Geometry: final body of the model. Coordinates: model frame, mm. Face numbers are marked on the shaded views. A direction names the side the tool comes from. Round coordinates to 2 decimals unless told otherwise and drop trailing zeros. Loops run counter-clockwise (first coordinate to the right, second up) from the corner with the lowest first, then second, coordinate; pieces in that order, holes last. Notation, with made-up numbers: M -25.5,82 L -8.5,82 A13 cw -8.5,92 Z; hole C 44.5,36 d8. An arc over 180 degrees is marked long. Write each question's results on one line, items separated by ' | '.
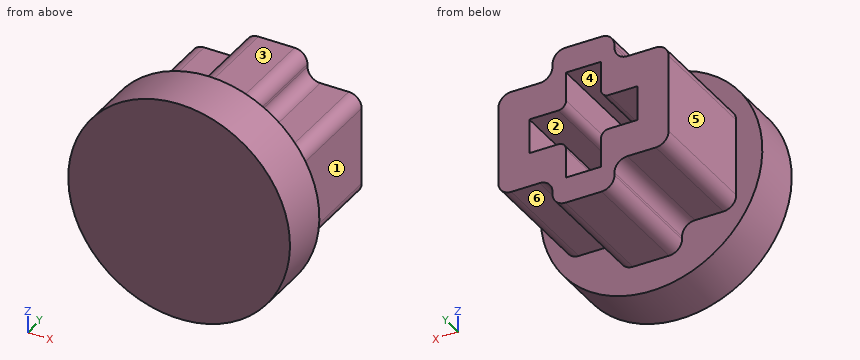
```python
from build123d import *

# Parameters (mm, degrees)
BUTTON_TOP_DEPTH        = 1.8
BUTTON_WALLS_DEPTH      = 4.8
OFFSET_2_DEPTH          = 0.2
STEM_START              = 0.2
STEM_HOUSING_DEPTH      = 4.6
SPOKES_DEPTH            = 0.2
CHAMFER1_SIZE           = 1.5
SKETCH11_R              = 47.776797093
SKETCH11_R_2            = 4.295081168
CUT_EXTRUDE1_DEPTH      = 10
CUT_EXTRUDE1_DEPTH_BACK = 10


with BuildPart() as part:
    # Sketch1 → button top (new body)
    with BuildSketch(Plane(origin=(0, 0, 0), x_dir=(1, 0, 0), z_dir=(0, 1, 0))):
        with BuildLine():
            Line((17, -12), (-17, -12))
            ThreePointArc((-17, -12), (-29, 0), (-17, 12))
            Line((-17, 12), (17, 12))
            ThreePointArc((17, 12), (29, 0), (17, -12))
        make_face()
    extrude(amount=BUTTON_TOP_DEPTH)

    # Sketch2 → button walls (add)
    with BuildSketch(Plane(origin=(0, 1.8, 0), x_dir=(1, 0, 0), z_dir=(0, 1, 0))):
        with BuildLine():
            Line((-17, 12), (17, 12))
            ThreePointArc((17, 12), (29, 0), (17, -12))
            Line((17, -12), (-17, -12))
            ThreePointArc((-17, -12), (-29, 0), (-17, 12))
        make_face()
        with BuildLine():
            Line((-17, 10.2), (17, 10.2))
            ThreePointArc((17, 10.2), (27.2, 0), (17, -10.2))
            Line((17, -10.2), (-17, -10.2))
            ThreePointArc((-17, -10.2), (-27.2, 0), (-17, 10.2))
        make_face(mode=Mode.SUBTRACT)
    extrude(amount=BUTTON_WALLS_DEPTH)

    # Sketch5 → offset 2 (add)
    with BuildSketch(Plane(origin=(0, 1.8, 0), x_dir=(1, 0, 0), z_dir=(0, 1, 0))):
        with BuildLine():
            Line((-12, 5), (12, 5))
            ThreePointArc((12, 5), (17, 0), (12, -5))
            Line((12, -5), (-12, -5))
            ThreePointArc((-12, -5), (-17, 0), (-12, 5))
        make_face()
    extrude(amount=OFFSET_2_DEPTH)

    # Sketch3 → stem housing (add)
    with BuildSketch(Plane(origin=(0, 1.8, 0), x_dir=(1, 0, 0), z_dir=(0, 1, 0)).offset(STEM_START)):
        with BuildLine():
            Line((-3.6, 2.6), (-3.6, -2.6))
            Line((-3.6, -2.6), (-1.496662955, -2.6))
            ThreePointArc((-1.496662955, -2.6), (0, -3), (1.496662955, -2.6))
            Line((1.496662955, -2.6), (3.6, -2.6))
            Line((3.6, -2.6), (3.6, 2.6))
            Line((3.6, 2.6), (1.496662955, 2.6))
            ThreePointArc((1.496662955, 2.6), (0, 3), (-1.496662955, 2.6))
            Line((-1.496662955, 2.6), (-3.6, 2.6))
        make_face()
        with BuildLine():
            Line((-0.675, 0.975), (-0.675, 2.1))
            Line((-0.675, 2.1), (0.675, 2.1))
            Line((0.675, 2.1), (0.675, 0.975))
            ThreePointArc((0.675, 0.975), (0.762867966, 0.762867966), (0.975, 0.675))
            Line((0.975, 0.675), (2.1, 0.675))
            Line((2.1, 0.675), (2.1, -0.675))
            Line((2.1, -0.675), (0.975, -0.675))
            ThreePointArc((0.975, -0.675), (0.762867966, -0.762867966), (0.675, -0.975))
            Line((0.675, -0.975), (0.675, -2.1))
            Line((0.675, -2.1), (-0.675, -2.1))
            Line((-0.675, -2.1), (-0.675, -0.975))
            ThreePointArc((-0.675, -0.975), (-0.762867966, -0.762867966), (-0.975, -0.675))
            Line((-0.975, -0.675), (-2.1, -0.675))
            Line((-2.1, -0.675), (-2.1, 0.675))
            Line((-2.1, 0.675), (-0.975, 0.675))
            ThreePointArc((-0.975, 0.675), (-0.762867966, 0.762867966), (-0.675, 0.975))
        make_face(mode=Mode.SUBTRACT)
        with BuildLine():
            ThreePointArc((14.738, -2), (15.091553391, -1.853553391), (15.238, -1.5))
            Line((15.238, -1.5), (15.238, 1.5))
            ThreePointArc((15.238, 1.5), (15.091553391, 1.853553391), (14.738, 2))
            Line((14.738, 2), (13.638, 2))
            ThreePointArc((13.638, 2), (13.284446609, 2.146446609), (13.138, 2.5))
            Line((13.138, 2.5), (13.138, 2.6))
            ThreePointArc((13.138, 2.6), (12.991553391, 2.953553391), (12.638, 3.1))
            Line((12.638, 3.1), (11.238, 3.1))
            ThreePointArc((11.238, 3.1), (10.884446609, 2.953553391), (10.738, 2.6))
            Line((10.738, 2.6), (10.738, 2.5))
            ThreePointArc((10.738, 2.5), (10.591553391, 2.146446609), (10.238, 2))
            Line((10.238, 2), (9.138, 2))
            ThreePointArc((9.138, 2), (8.784446609, 1.853553391), (8.638, 1.5))
            Line((8.638, 1.5), (8.638, -1.5))
            ThreePointArc((8.638, -1.5), (8.784446609, -1.853553391), (9.138, -2))
            Line((9.138, -2), (10.238, -2))
            ThreePointArc((10.238, -2), (10.591553391, -2.146446609), (10.738, -2.5))
            Line((10.738, -2.5), (10.738, -2.6))
            ThreePointArc((10.738, -2.6), (10.884446609, -2.953553391), (11.238, -3.1))
            Line((11.238, -3.1), (12.638, -3.1))
            ThreePointArc((12.638, -3.1), (12.991553391, -2.953553391), (13.138, -2.6))
            Line((13.138, -2.6), (13.138, -2.5))
            ThreePointArc((13.138, -2.5), (13.284446609, -2.146446609), (13.638, -2))
            Line((13.638, -2), (14.738, -2))
        make_face()
        with BuildLine():
            Line((14.038, 0.675), (14.038, -0.675))
            Line((14.038, -0.675), (12.913, -0.675))
            ThreePointArc((12.913, -0.675), (12.700867966, -0.762867966), (12.613, -0.975))
            Line((12.613, -0.975), (12.613, -2.1))
            Line((12.613, -2.1), (11.263, -2.1))
            Line((11.263, -2.1), (11.263, -0.975))
            ThreePointArc((11.263, -0.975), (11.175132034, -0.762867966), (10.963, -0.675))
            Line((10.963, -0.675), (9.838, -0.675))
            Line((9.838, -0.675), (9.838, 0.675))
            Line((9.838, 0.675), (10.963, 0.675))
            ThreePointArc((10.963, 0.675), (11.175132034, 0.762867966), (11.263, 0.975))
            Line((11.263, 0.975), (11.263, 2.1))
            Line((11.263, 2.1), (12.613, 2.1))
            Line((12.613, 2.1), (12.613, 0.975))
            ThreePointArc((12.613, 0.975), (12.700867966, 0.762867966), (12.913, 0.675))
            Line((12.913, 0.675), (14.038, 0.675))
        make_face(mode=Mode.SUBTRACT)
        with BuildLine():
            Line((-13.138, 2.6), (-13.138, 2.5))
            ThreePointArc((-13.138, 2.5), (-13.284446609, 2.146446609), (-13.638, 2))
            Line((-13.638, 2), (-14.738, 2))
            ThreePointArc((-14.738, 2), (-15.091553391, 1.853553391), (-15.238, 1.5))
            Line((-15.238, 1.5), (-15.238, -1.5))
            ThreePointArc((-15.238, -1.5), (-15.091553391, -1.853553391), (-14.738, -2))
            Line((-14.738, -2), (-13.638, -2))
            ThreePointArc((-13.638, -2), (-13.284446609, -2.146446609), (-13.138, -2.5))
            Line((-13.138, -2.5), (-13.138, -2.6))
            ThreePointArc((-13.138, -2.6), (-12.991553391, -2.953553391), (-12.638, -3.1))
            Line((-12.638, -3.1), (-11.238, -3.1))
            ThreePointArc((-11.238, -3.1), (-10.884446609, -2.953553391), (-10.738, -2.6))
            Line((-10.738, -2.6), (-10.738, -2.5))
            ThreePointArc((-10.738, -2.5), (-10.591553391, -2.146446609), (-10.238, -2))
            Line((-10.238, -2), (-9.138, -2))
            ThreePointArc((-9.138, -2), (-8.784446609, -1.853553391), (-8.638, -1.5))
            Line((-8.638, -1.5), (-8.638, 1.5))
            ThreePointArc((-8.638, 1.5), (-8.784446609, 1.853553391), (-9.138, 2))
            Line((-9.138, 2), (-10.238, 2))
            ThreePointArc((-10.238, 2), (-10.591553391, 2.146446609), (-10.738, 2.5))
            Line((-10.738, 2.5), (-10.738, 2.6))
            ThreePointArc((-10.738, 2.6), (-10.884446609, 2.953553391), (-11.238, 3.1))
            Line((-11.238, 3.1), (-12.638, 3.1))
            ThreePointArc((-12.638, 3.1), (-12.991553391, 2.953553391), (-13.138, 2.6))
        make_face()
        with BuildLine():
            ThreePointArc((-12.913, 0.675), (-12.700867966, 0.762867966), (-12.613, 0.975))
            Line((-12.613, 0.975), (-12.613, 2.1))
            Line((-12.613, 2.1), (-11.263, 2.1))
            Line((-11.263, 2.1), (-11.263, 0.975))
            ThreePointArc((-11.263, 0.975), (-11.175132034, 0.762867966), (-10.963, 0.675))
            Line((-10.963, 0.675), (-9.838, 0.675))
            Line((-9.838, 0.675), (-9.838, -0.675))
            Line((-9.838, -0.675), (-10.963, -0.675))
            ThreePointArc((-10.963, -0.675), (-11.175132034, -0.762867966), (-11.263, -0.975))
            Line((-11.263, -0.975), (-11.263, -2.1))
            Line((-11.263, -2.1), (-12.613, -2.1))
            Line((-12.613, -2.1), (-12.613, -0.975))
            ThreePointArc((-12.613, -0.975), (-12.700867966, -0.762867966), (-12.913, -0.675))
            Line((-12.913, -0.675), (-14.038, -0.675))
            Line((-14.038, -0.675), (-14.038, 0.675))
            Line((-14.038, 0.675), (-12.913, 0.675))
        make_face(mode=Mode.SUBTRACT)
    extrude(amount=STEM_HOUSING_DEPTH)

    # Sketch4 → spokes (add)
    with BuildSketch(Plane(origin=(0, 1.8, 0), x_dir=(1, 0, 0), z_dir=(0, 1, 0))):
        with BuildLine():
            Line((-0.8, 3), (-0.8, 10.2))
            ThreePointArc((-0.8, 10.2), (0, 11), (0.8, 10.2))
            Line((0.8, 10.2), (0.8, 3))
            ThreePointArc((0.8, 3), (0, 2.2), (-0.8, 3))
        make_face()
        with BuildLine():
            Line((17, -0.8), (27.2, -0.8))
            ThreePointArc((27.2, -0.8), (28, 0), (27.2, 0.8))
            Line((27.2, 0.8), (17, 0.8))
            ThreePointArc((17, 0.8), (16.2, 0), (17, -0.8))
        make_face()
        with BuildLine():
            Line((11.2, 3.1), (11.2, 10.2))
            ThreePointArc((11.2, 10.2), (12, 11), (12.8, 10.2))
            Line((12.8, 10.2), (12.8, 3.1))
            ThreePointArc((12.8, 3.1), (12, 2.3), (11.2, 3.1))
        make_face()
        with BuildLine():
            Line((-12.8, 3.1), (-12.8, 10.2))
            ThreePointArc((-12.8, 10.2), (-12, 11), (-11.2, 10.2))
            Line((-11.2, 10.2), (-11.2, 3.1))
            ThreePointArc((-11.2, 3.1), (-12, 2.3), (-12.8, 3.1))
        make_face()
        with BuildLine():
            Line((-17, -0.8), (-27.2, -0.8))
            ThreePointArc((-27.2, -0.8), (-28, 0), (-27.2, 0.8))
            Line((-27.2, 0.8), (-17, 0.8))
            ThreePointArc((-17, 0.8), (-16.2, 0), (-17, -0.8))
        make_face()
        with BuildLine():
            Line((-0.8, -3), (-0.8, -10.2))
            ThreePointArc((-0.8, -10.2), (0, -11), (0.8, -10.2))
            Line((0.8, -10.2), (0.8, -3))
            ThreePointArc((0.8, -3), (0, -2.2), (-0.8, -3))
        make_face()
        with BuildLine():
            Line((11.2, -3.1), (11.2, -10.2))
            ThreePointArc((11.2, -10.2), (12, -11), (12.8, -10.2))
            Line((12.8, -10.2), (12.8, -3.1))
            ThreePointArc((12.8, -3.1), (12, -2.3), (11.2, -3.1))
        make_face()
        with BuildLine():
            Line((-12.8, -3.1), (-12.8, -10.2))
            ThreePointArc((-12.8, -10.2), (-12, -11), (-11.2, -10.2))
            Line((-11.2, -10.2), (-11.2, -3.1))
            ThreePointArc((-11.2, -3.1), (-12, -2.3), (-12.8, -3.1))
        make_face()
    extrude(amount=SPOKES_DEPTH)

    # Chamfer1
    chamfer1_edges = [part.edges().sort_by_distance(p)[0] for p in [
        (-27.2, 6.6, 0),
        (0, 6.6, 10.2),
        (27.2, 6.6, 0),
        (0, 6.6, -10.2),
    ]]
    chamfer(chamfer1_edges, length=CHAMFER1_SIZE)

    # Cut-Sweep1: sweep along a path in Sketch10
    with BuildLine(Plane.XZ) as cut_sweep1_path:
        Line((-17, 12), (17, 12))
        ThreePointArc((17, 12), (29, 0), (17, -12))
        Line((17, -12), (-17, -12))
        ThreePointArc((-17, -12), (-29, 0), (-17, 12))
    # Sketch6 → Cut-Sweep1 (sweep, cut)
    with BuildSketch(Plane.XY):
        with BuildLine():
            Line((-28.261522369, 0), (-28.461522369, 0.2))
            ThreePointArc((-28.461522369, 0.2), (-28.860054223, 0.79644507), (-29, 1.5))
            Line((-29, 1.5), (-29, 0))
            Line((-29, 0), (-28.261522369, 0))
        make_face()
    sweep(path=cut_sweep1_path.line, mode=Mode.SUBTRACT)

    # Sketch11 → Cut-Extrude1 (cut, two sides)
    with BuildSketch(Plane(origin=(0, 2, 0), x_dir=(1, 0, 0), z_dir=(0, 1, 0))) as cut_extrude1_sk:
        with Locations((-11.954336916, 0)):
            Circle(SKETCH11_R)
        with Locations(Location((-11.954336916, 0, 0), (0, 0, 270))):
            Circle(SKETCH11_R_2, mode=Mode.SUBTRACT)
    extrude(amount=CUT_EXTRUDE1_DEPTH, mode=Mode.SUBTRACT)
    extrude(cut_extrude1_sk.sketch, amount=-CUT_EXTRUDE1_DEPTH_BACK, mode=Mode.SUBTRACT)


solid = part.part
```
1. Section C-C (x = -13.25). Output: boundary loops of the cut face in (y, z) (3 decimals), then the cut area to 3 significant figures.
Answer key:
outline: M 0,-4.095 L 2,-4.095 L 2,-2.185 L 6.6,-2.185 L 6.6,-0.675 L 2,-0.675 L 2,0.675 L 6.6,0.675 L 6.6,2.185 L 2,2.185 L 2,4.095 L 0,4.095 Z | area: 30.3 mm²
2. Pin query (flat end, axial travel): P1, Ø1.1, axis at x = -12, y = 4.5, coming from the -Z side; P2, Ø2.5, axis at y = 5, z = 0, coming from the -X side; P3, Ø1.5, axis at y = 1.5, z = 1.5, coming from the +X side. Return the tip coordinate at first contact, or that it passes through.
Answer key:
P1: stops at z = -3.1 | P2: stops at x = -15.24 | P3: stops at x = -7.73
3. Section B-B (x = -8.75). Output: boundary loops of the cut face in (y, z).
Answer key:
outline: M 0,-2.86 L 2,-2.86 L 2,-1.82 L 6.6,-1.82 L 6.6,1.82 L 2,1.82 L 2,2.86 L 0,2.86 Z
4. Section D-D (z = 2.25). Output: boundary loops of the cut face in (x, y), then the cut area to 3 significant figures.
Answer key:
outline: M -15.61,0 L -8.3,0 L -8.3,2 L -10.67,2 L -10.67,6.6 L -13.2,6.6 L -13.2,2 L -15.61,2 Z | area: 26.3 mm²
5. Draft query along Z for the marked faces 1, 2 and 3. Return one class per face: pulls with the +Z half, pulls with the -Z half, needs draft (parallel to the pull), parting line crosses it, or undercut.
Answer key:
face 1: needs draft | face 2: undercut | face 3: pulls with the +Z half
6. Access query for the marked faces 4, 5 and 6. Directions: +Z, -Z, +X, -X, +Y, -Y. A direction counts if a zero-diameter tool reaches every point of the face in a straight line with its end or side. Return the directions, or none.
Answer key:
face 4: +Y | face 5: +Z, -Z, -X, +Y | face 6: -Z, +X, +Y
7. Section A-A (z = 0). Output: boundary loops of the cut face in (x, y), then the cut area to 3 significant figures.
Answer key:
outline: M -16.25,0 L -7.66,0 L -7.66,2 L -8.64,2 L -8.64,6.6 L -9.84,6.6 L -9.84,2 L -14.04,2 L -14.04,6.6 L -15.24,6.6 L -15.24,2 L -16.25,2 Z | area: 28.2 mm²
8. Ray query, probe 1 along X at (y, z) = (4.75, 0.5); probe 2 along Y at (x, z) = (-8.5, 1); probe 3 along X at (y, z) = (4, -0.75). Return the intervals inside material, ascending.
Answer key:
probe 1: x = -15.24 to -14.04, -9.84 to -8.64 | probe 2: y = 0 to 2 | probe 3: x = -15.24 to -12.71, -11.16 to -8.64
